from build123d import *

# Parameters (mm, degrees)
SKETCH1_W           = 56.35
SKETCH1_H           = 85
BOSS_EXTRUDE1_DEPTH = 55.5
CUT_EXTRUDE3_DEPTH  = 117.105867638
CUT_EXTRUDE4_DEPTH  = 18
SKETCH2_4_W         = 10.275
SKETCH2_4_H         = 15.5
SKETCH2_4_W_2       = 4.725
SKETCH2_4_W_3       = 15
SKETCH2_4_W_4       = 6.075
SKETCH2_4_H_2       = 13.5
SKETCH2_4_W_5       = 9.825
BOSS_EXTRUDE2_DEPTH = 3
SKETCH3_W           = 6.5
SKETCH3_H           = 52.5
BOSS_EXTRUDE3_DEPTH = 2.4
SKETCH4_W           = 83.236605227
SKETCH4_H           = 41.384754339
CUT_EXTRUDE5_DEPTH  = 117.105867638
SKETCH6_W           = 56.35
SKETCH6_H           = 69.665906653
BOSS_EXTRUDE4_DEPTH = 13.5
SKETCH5_R           = 1.5
CUT_EXTRUDE6_DEPTH  = 104.924600071
SKETCH7_W           = 101.583675899
SKETCH7_H           = 36.04582048
CUT_EXTRUDE7_DEPTH  = 5


with BuildPart() as part:
    # Sketch1 → Boss-Extrude1 (new body)
    with BuildSketch(Plane.XY):
        with Locations((28.175, 42.5)):
            Rectangle(SKETCH1_W, SKETCH1_H)
    extrude(amount=BOSS_EXTRUDE1_DEPTH)

    # Sketch2 → Cut-Extrude3 (cut, through all)
    with BuildSketch(Plane.XZ):
        with BuildLine():
            Line((5.575, 25.1), (0, 25.1))
            Line((0, 25.1), (0, 0))
            Line((0, 0), (11.575, 0))
            ThreePointArc((11.575, 0), (7.332359313, 1.757359313), (5.575, 6))
            Line((5.575, 6), (5.575, 25.1))
        make_face()
        with BuildLine():
            Line((56.35, 0), (56.35, 25.1))
            Line((56.35, 25.1), (50.775, 25.1))
            Line((50.775, 25.1), (50.775, 6))
            ThreePointArc((50.775, 6), (49.017640687, 1.757359313), (44.775, 0))
            Line((44.775, 0), (56.35, 0))
        make_face()
        Polygon((56.35, 55.5), (44.175, 55.5), (44.175, 50.5), (54, 50.5), (54, 37), (56.35, 37), align=None)
        Polygon((1.9, 37), (1.9, 52.5), (12.175, 52.5), (12.175, 55.5), (0, 55.5), (0, 37), align=None)
    extrude(amount=-CUT_EXTRUDE3_DEPTH, mode=Mode.SUBTRACT)

    # Sketch2<3> → Cut-Extrude4 (cut)
    with BuildSketch(Plane.XZ):
        Polygon((12.175, 55.5), (12.175, 52.5), (16.9, 52.5), (16.9, 37), (20.05, 37), (20.05, 52.5), (35.05, 52.5), (35.05, 37), (38.1, 37), (38.1, 50.5), (44.175, 50.5), (44.175, 55.5), align=None)
    extrude(amount=-CUT_EXTRUDE4_DEPTH, mode=Mode.SUBTRACT)

    # Sketch2<4> → Boss-Extrude2 (add)
    with BuildSketch(Plane.XZ):
        with Locations((7.0375, 44.75)):
            Rectangle(SKETCH2_4_W, SKETCH2_4_H)
        with Locations((14.5375, 44.75)):
            Rectangle(SKETCH2_4_W_2, SKETCH2_4_H)
        with Locations((27.55, 44.75)):
            Rectangle(SKETCH2_4_W_3, SKETCH2_4_H)
        with Locations((41.1375, 43.75)):
            Rectangle(SKETCH2_4_W_4, SKETCH2_4_H_2)
        with Locations((49.0875, 43.75)):
            Rectangle(SKETCH2_4_W_5, SKETCH2_4_H_2)
    extrude(amount=BOSS_EXTRUDE2_DEPTH)

    # Sketch3 → Boss-Extrude3 (add)
    with BuildSketch(Plane.ZY.offset(-1.9)):
        with Locations((40.25, 53.45)):
            Rectangle(SKETCH3_W, SKETCH3_H)
        with Locations((29.75, 53.45)):
            Rectangle(SKETCH3_W, SKETCH3_H)
    extrude(amount=BOSS_EXTRUDE3_DEPTH)

    # Sketch4 → Cut-Extrude5 (cut, through all)
    with BuildSketch(Plane.XZ):
        with Locations((28.392096551, 14.80762283)):
            Rectangle(SKETCH4_W, SKETCH4_H)
    extrude(amount=-CUT_EXTRUDE5_DEPTH, mode=Mode.SUBTRACT)

    # Sketch6 → Boss-Extrude4 (add)
    with BuildSketch(Plane.XY.offset(50.5)):
        with Locations((28.175, 50.167046674)):
            Rectangle(SKETCH6_W, SKETCH6_H)
    extrude(amount=-BOSS_EXTRUDE4_DEPTH)

    # Sketch5 → Cut-Extrude6 (cut, through all)
    with BuildSketch(Plane(origin=(0, 0, 35.5), x_dir=(-1, 0, 0), z_dir=(0, 0, -1))):
        with Locations((-52.675, 81.6)):
            Circle(SKETCH5_R)
        with Locations((-3.675, 81.6)):
            Circle(SKETCH5_R)
        with Locations((-3.675, 23.6)):
            Circle(SKETCH5_R)
        with Locations((-52.675, 23.6)):
            Circle(SKETCH5_R)
    extrude(amount=-CUT_EXTRUDE6_DEPTH, mode=Mode.SUBTRACT)

    # Sketch7 → Cut-Extrude7 (cut)
    with BuildSketch(Plane.XY.offset(55.5)):
        with Locations((37.583210273, 98.02291024)):
            Rectangle(SKETCH7_W, SKETCH7_H)
    extrude(amount=-CUT_EXTRUDE7_DEPTH, mode=Mode.SUBTRACT)


solid = part.part
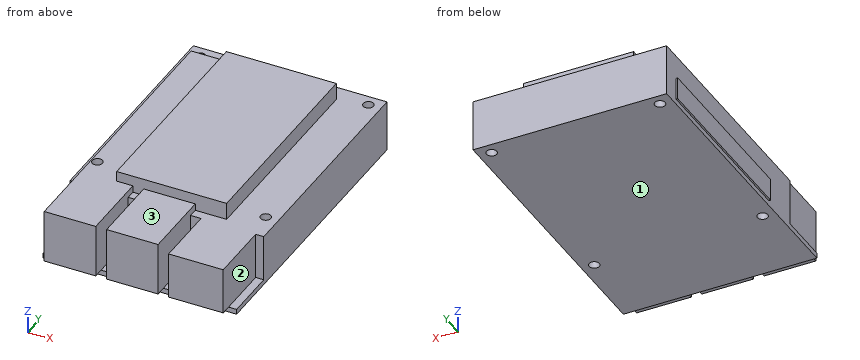
Design review of the part built by this model. Coordinates are the model's own, in mm. Face numbers are marked on the shaded views. A direction names the side the tool comes from. Round coordinates to 2 decimals unless told otherwise and drop trailing zeros. Write each loop counter-clockwise with the first axis right and the second up, starting at its lowest first coordinate (ties: lowest second). Pieces come first, ordered by that corner, then holes. Notation, with made-up numbers: (53.25, 52) - (109.25, 52) arc R11 ccw to (109.25, 63) - close; hole circle Ø2 at (31.5, 43.5). An arc over 180 degrees is marked (long way). Use a Markdown table: item, result. Add a question column.
1. Clearance check with flat-ended pins moving along their axes: pin 1 (2 mm diameter, centred on y = 65.5, z = 53, fed in from -X); pin 2 (5.5 mm diameter, centred on x = 29.5, z = 54, fed in from +Y); pin 3 (0.6 mm diameter, centred on x = -0.5, y = 49, fed in from +Z). State where each tip first meets the part, or that it passes through.
2. We need section B-B (z = 48). State the section outline as (x, y) points (3 decimals).
3. Wall thickness on probe 1 along X at (y, z) = (81.6, 42) (3 decimals); probe 2 along X at (y, z) = (4, 37.5); probe 3 along Y at (x, z) = (15, 51): over which ranges is each line inside the solid? List them lowest first.
4. For the marked faces 1, 2 and 3, list the 3-axis set-ups (+Z, -Z, +X, -X, +Y, -Y) from which the entire face can be reached by the end or side of a thin tool; tool diameter is ignored.
5. We need section D-D (y = 23.6). State the section outline as (x, z) points (3 decimals).
6. We need section C-C (x = 21). State the section outline as (y, z) points, then the cut area to 3 significant figures.
7. We need section A-A (y = 81.6). State the section outline as (x, z) points (3 decimals), then the cut area to 3 significant figures.
Output:
| question | item | result |
|---|---|---|
| 1 | pin 1 | stops at x = 1.9 |
| 1 | pin 2 | stops at y = 80 |
| 1 | pin 3 | stops at z = 43.5 |
| 2 | outline | (0, 15.334) - (1.9, 15.334) - (1.9, -3) - (16.9, -3) - (16.9, 15.334) - (20.05, 15.334) - (20.05, -3) - (35.05, -3) - (35.05, 15.334) - (38.1, 15.334) - (38.1, -3) - (54, -3) - (54, 15.334) - (56.35, 15.334) - (56.35, 85) - (0, 85) - close; hole circle Ø3 at (3.675, 23.6); hole circle Ø3 at (3.675, 81.6); hole circle Ø3 at (52.675, 23.6); hole circle Ø3 at (52.675, 81.6) |
| 3 | probe 1 | x = 0 to 2.175, 5.175 to 51.175, 54.175 to 56.35 |
| 3 | probe 2 | x = 1.9 to 16.9, 20.05 to 35.05, 38.1 to 54 |
| 3 | probe 3 | y = -3 to 80 |
| 4 | face 1 | -Z, +X, -X, +Y, -Y |
| 4 | face 2 | +Z, +X, -Y |
| 4 | face 3 | +Z, +X, -X, -Y |
| 5 | outline | (0, 35.5) - (2.175, 35.5) - (2.175, 52.5) - (1.9, 52.5) - (1.9, 50.5) - (0, 50.5) - close; (5.175, 35.5) - (51.175, 35.5) - (51.175, 50.5) - (44.175, 50.5) - (44.175, 55.5) - (12.175, 55.5) - (12.175, 52.5) - (5.175, 52.5) - close; (54.175, 35.5) - (56.35, 35.5) - (56.35, 50.5) - (54.175, 50.5) - close |
| 6 | outline | (-3, 37) - (0, 37) - (0, 35.5) - (85, 35.5) - (85, 50.5) - (80, 50.5) - (80, 55.5) - (18, 55.5) - (18, 52.5) - (-3, 52.5) - close |
| 6 | area | 1,670 mm2 |
| 7 | outline | (0, 35.5) - (2.175, 35.5) - (2.175, 50.5) - (0, 50.5) - close; (5.175, 35.5) - (51.175, 35.5) - (51.175, 50.5) - (5.175, 50.5) - close; (54.175, 35.5) - (56.35, 35.5) - (56.35, 50.5) - (54.175, 50.5) - close |
| 7 | area | 755 mm2 |
